Read the model definition and answer for the solid it produces. Units are mm, in the model's axes. A direction names the side the tool comes from. Round coordinates to 2 decimals unless told otherwise and drop trailing zeros. Order: outer loops, then holes, each group sorted by start corner. A loop starts at its lowest first (then second) coordinate and runs counter-clockwise, first axis right, second up. Notation, with made-up numbers: (-34, 6) - (22, 6) arc R6 ccw to (22, 11) - close; hole circle Ø10 at (74.5, 12.5). An arc over 180 degrees is marked (long way). Put each result on its own line as item: value. Start each with the question number.
Q1. Find the intervals of material crossed by line 1 along X through (y, z) = (5, 35.5); line 2 along Z through (x, y) = (29.5, 9); line 3 along Y through (x, z) = (14.5, 6), in increasing order. Write a range as from..to.
Q2. Which of the six approach directions +Z, -Z, +X, -X, +Y, -Y give full straight-line access (tool end or side, diameter ignored) to faces 4 (the face through (40, 23, 16)), 5 (the face through (10, 15, 28)), 6 (the face through (20, 50, 7))?
Q3. For a pull along X with two mould halves and no side action, classify faces 1 (the face through (0, 23, 16)), 2 (the face through (20, 30, 0)), 3 (the face through (30, 15, 28)) as pulls with the +X half, pulls with the -X half, needs draft (parallel to the pull), parting line crosses it, or undercut.
Q4. Section A-A on y = 56.5 is taken. Give the vertices of the cut face in (x, z), then the cut area to 3 significant figures.
Q5. Each of these flat-tipped pins is pushed along its axis until it touches: pin 1 Ø1 at (x, z) = (11.5, 20) entering from -Y; pin 2 Ø16.5 at (x, z) = (20, 7.5) entering from +Y; pin 3 Ø10 at (x, y) = (29, 43) entering from +Z; pin 4 Ø4 at (x, y) = (35.5, 29) entering from +Z. Where does it stop, or does it pass through?
Q6. Section C-C on z = 5.5 is taken. Give the vertices of the cut face in (x, y).
Q7. Section D-D on y = 9.5 is taken. Give the vertices of the cut face in (x, z), then the cut area to 4 significant figures.
Q8. Section B-B on z = 26 is taken. Give the vertices of the cut face in (x, y).
from build123d import *

# Parameters (mm, degrees)
F1_DEPTH = 40
F2_W     = 20
F2_H     = 10
F3_DEPTH = 40.001
F4_W     = 20
F4_H     = 20
F5_DEPTH = 60.001


with BuildPart() as f1:
    # F0 (on Right) → F1 (new body)
    with BuildSketch(Plane.YZ):
        Polygon((60, 10), (0, 40), (0, 0), (60, 0), align=None)
    extrude(amount=F1_DEPTH)

    # F2 (on face) → F3 (cut, through all)
    with BuildSketch(Plane(origin=(0, 0, 0), x_dir=(1, 0, 0), z_dir=(0, 0, -1))):
        with Locations((20, -55)):
            Rectangle(F2_W, F2_H)
    extrude(amount=-F3_DEPTH, mode=Mode.SUBTRACT)

    # F4 (on face) → F5 (cut, through all)
    with BuildSketch(Plane.XZ):
        with Locations((20, 30)):
            Rectangle(F4_W, F4_H)
    extrude(amount=-F5_DEPTH, mode=Mode.SUBTRACT)


solid = f1.part
Findings:
1. line 1: 0..10, 30..40
1. line 2: 0..20
1. line 3: 0..50
2. face 4: +Z, -Z, +X, +Y, -Y
2. face 5: +Z, +Y, -Y
2. face 6: +Z, -Z, +Y
3. face 1: pulls with the -X half
3. face 2: needs draft
3. face 3: undercut
4. outline: (0, 0) - (10, 0) - (10, 11.75) - (0, 11.75) - close; (30, 0) - (40, 0) - (40, 11.75) - (30, 11.75) - close
4. area: 235 mm2
5. pin 1: y = 0
5. pin 2: y = 50
5. pin 3: z = 20.95
5. pin 4: z = 26.5
6. outline: (0, 0) - (40, 0) - (40, 60) - (30, 60) - (30, 50) - (10, 50) - (10, 60) - (0, 60) - close
7. outline: (0, 0) - (40, 0) - (40, 35.25) - (30, 35.25) - (30, 20) - (10, 20) - (10, 35.25) - (0, 35.25) - close
7. area: 1,105 mm2
8. outline: (0, 0) - (10, 0) - (10, 28) - (0, 28) - close; (30, 0) - (40, 0) - (40, 28) - (30, 28) - close
